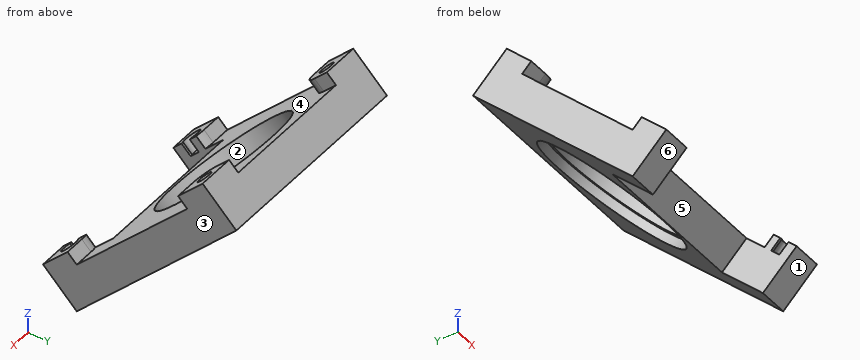
```python
from build123d import *
from OCP.BRepAlgoAPI import BRepAlgoAPI_Cut
from OCP.TopTools import TopTools_ListOfShape

# Parameters (mm, degrees)
SKETCH3_W               = 37
SKETCH3_H               = 39
SKETCH3_R               = 12
BOSS_EXTRUDE1_DEPTH     = 4.5
SKETCH4_W               = 37
SKETCH4_H               = 39
SKETCH4_R               = 13
BOSS_EXTRUDE2_DEPTH     = 1.5
SKETCH5_R               = 1.25
BOSS_EXTRUDE4_DEPTH     = 2.238877686
CUT_EXTRUDE1_DEPTH      = 3
CUT_EXTRUDE1_DEPTH_BACK = 7.261122
SKETCH7_W               = 27
SKETCH7_H               = 10


with BuildPart() as part:
    # Sketch3 → Boss-Extrude1 (new body)
    with BuildSketch(Plane(origin=(0, -51.218608926, 51.218608926), x_dir=(1, 0, 0), z_dir=(-2.4581031654591364e-15, -0.7071067811865478, 0.7071067811865472))):
        with Locations((73.844609768, 127.312236852)):
            Rectangle(SKETCH3_W, SKETCH3_H)
        with Locations(Location((73.844609768, 131.312236852, 0), (0, 0, 270))):
            Circle(SKETCH3_R, mode=Mode.SUBTRACT)
    extrude(amount=-BOSS_EXTRUDE1_DEPTH)

    # Sketch4 → Boss-Extrude2 (add)
    with BuildSketch(Plane(origin=(0, -48.036628411, 48.036628411), x_dir=(1, 0, 0), z_dir=(2.4581031654591364e-15, 0.7071067811865478, -0.7071067811865472))):
        with Locations((73.844609768, -127.312236852)):
            Rectangle(SKETCH4_W, SKETCH4_H)
        with Locations(Location((73.844609768, -131.312236852, 0), (0, 0, 90))):
            Circle(SKETCH4_R, mode=Mode.SUBTRACT)
    extrude(amount=BOSS_EXTRUDE2_DEPTH)

    # Sketch5 → Boss-Extrude4 (add)
    # profile 1 of 4: a face of its own
    with BuildSketch(Plane(origin=(0, -51.218608926, 51.218608926), x_dir=(1, 0, 0), z_dir=(-2.386964886512496e-15, -0.7071067811865477, 0.7071067811865475))):
        with BuildLine():
            Line((92.344609768, 107.812236852), (92.344609768, 113.812236852))
            Line((92.344609768, 113.812236852), (88.844609768, 113.812236852))
            ThreePointArc((88.844609768, 113.812236852), (88.068152632, 113.710014331), (87.344609768, 113.410313064))
            Line((87.344609768, 113.410313064), (87.344609768, 111.807298734))
            Line((87.344609768, 111.807298734), (87.722178544, 111.807298734))
            ThreePointArc((87.722178544, 111.807298734), (90.344606124, 110.815542933), (87.726575779, 109.812236852))
            Line((87.726575779, 109.812236852), (87.344609768, 109.812236852))
            Line((87.344609768, 109.812236852), (87.344609768, 107.812236852))
            Line((87.344609768, 107.812236852), (92.344609768, 107.812236852))
        make_face()
    # profile 2 of 4: a face of its own
    with BuildSketch(Plane(origin=(0, -51.218608926, 51.218608926), x_dir=(1, 0, 0), z_dir=(-2.386964886512496e-15, -0.7071067811865477, 0.7071067811865475))):
        with BuildLine():
            Line((55.344609768, 107.812236852), (60.344609768, 107.812236852))
            Line((60.344609768, 107.812236852), (60.344609768, 109.812236852))
            Line((60.344609768, 109.812236852), (59.962643756, 109.812236852))
            ThreePointArc((59.962643756, 109.812236852), (57.344609768, 110.812236852), (59.962643756, 111.812236852))
            Line((59.962643756, 111.812236852), (60.344609768, 111.812236852))
            Line((60.344609768, 111.812236852), (60.344609768, 113.410313064))
            ThreePointArc((60.344609768, 113.410313064), (59.621066903, 113.710014331), (58.844609768, 113.812236852))
            Line((58.844609768, 113.812236852), (55.344609768, 113.812236852))
            Line((55.344609768, 113.812236852), (55.344609768, 107.812236852))
        make_face()
    # profile 3 of 4: a face of its own
    with BuildSketch(Plane(origin=(0, -51.218608926, 51.218608926), x_dir=(1, 0, 0), z_dir=(-2.386964886512496e-15, -0.7071067811865477, 0.7071067811865475))):
        with BuildLine():
            Line((55.344609768, 146.812236852), (55.344609768, 140.812236852))
            Line((55.344609768, 140.812236852), (58.844609768, 140.812236852))
            ThreePointArc((58.844609768, 140.812236852), (60.965930111, 141.690916509), (61.844609768, 143.812236852))
            Line((61.844609768, 143.812236852), (61.844609768, 146.812236852))
            Line((61.844609768, 146.812236852), (55.344609768, 146.812236852))
        make_face()
        with Locations(Location((58.844609768, 143.812236852, 0), (0, 0, 90))):
            Circle(SKETCH5_R, mode=Mode.SUBTRACT)
    # profile 4 of 4: a face of its own
    with BuildSketch(Plane(origin=(0, -51.218608926, 51.218608926), x_dir=(1, 0, 0), z_dir=(-2.386964886512496e-15, -0.7071067811865477, 0.7071067811865475))):
        with BuildLine():
            Line((92.344609768, 146.812236852), (85.844609768, 146.812236852))
            Line((85.844609768, 146.812236852), (85.844609768, 143.812236852))
            ThreePointArc((85.844609768, 143.812236852), (86.723289424, 141.690916509), (88.844609768, 140.812236852))
            Line((88.844609768, 140.812236852), (92.344609768, 140.812236852))
            Line((92.344609768, 140.812236852), (92.344609768, 146.812236852))
        make_face()
        with Locations(Location((88.844609768, 143.812236852, 0), (0, 0, 90))):
            Circle(SKETCH5_R, mode=Mode.SUBTRACT)
    extrude(amount=BOSS_EXTRUDE4_DEPTH)


with BuildPart() as cut_extrude1_tool:
    # Sketch7 → Cut-Extrude1 (new, two sides: drawn at the far end of the back side and taken through both)
    with BuildSketch(Plane(origin=(0, -46.084220099, 46.084220099), x_dir=(1, 0, 0), z_dir=(0, 0.7071067811865502, -0.7071067811865449)).offset(-CUT_EXTRUDE1_DEPTH_BACK)):
        with Locations((73.844609768, -112.812236852)):
            Rectangle(SKETCH7_W, SKETCH7_H)
    extrude(amount=CUT_EXTRUDE1_DEPTH + CUT_EXTRUDE1_DEPTH_BACK)


with BuildPart() as part_1:
    add(part.part)

    # Cut-Extrude1: cut by cut_extrude1_tool, with a tolerance
    cut_extrude1_stock = TopTools_ListOfShape()
    cut_extrude1_stock.Append(part_1.part.wrapped)
    cut_extrude1_tools = TopTools_ListOfShape()
    cut_extrude1_tools.Append(cut_extrude1_tool.part.wrapped)
    cut_extrude1_cut = BRepAlgoAPI_Cut()
    cut_extrude1_cut.SetArguments(cut_extrude1_stock)
    cut_extrude1_cut.SetTools(cut_extrude1_tools)
    cut_extrude1_cut.SetFuzzyValue(0.00001)
    cut_extrude1_cut.Build()
    add(Compound.cast(cut_extrude1_cut.Shape()).solids(), mode=Mode.REPLACE)


solid = part_1.part
```
Source: CAD feature listing. Evaluate the final solid. Frame: model axes, mm. Face numbers are marked on the shaded views. A direction names the side the tool comes from. Coordinates: 2 decimals unless noted, no trailing zeros. Loops run counter-clockwise (first coordinate to the right, second up) from the corner with the lowest first, then second, coordinate; pieces in that order, holes last. Notation, with made-up numbers: M 32,8 L 74,8 A25 cw 74,30 Z; hole C 27.5,10.5 d10. An arc over 180 degrees is marked long. Put each result on its own line as item: value. Start each with the question number.
1) Reachability of the marked faces 5 and 6 from +Z, -Z, +X, -X, +Y, -Y: full face, straight path, thin tool, end or side. Return the list, or none.
2) Cut plane D-D on x = 89.5. Return the cut outline in (y, z) (1 decimal), then the cut area to 3 significant figures.
3) Pull-direction query (X, two-part tool) for the marked faces 1, 2, 3 and 4; classes: pulls with the +X half, pulls with the -X half, needs draft (parallel to the pull), parting line crosses it, or undercut.
4) Cut plane B-B on z = 125.5. Return the cut outline in (x, y).
5) Contact query for flat-ended pins moving along their axis: pin 1 Ø3 at (x, z) = (71, 151) entering from -Y; pin 2 Ø12 at (x, z) = (77, 147) entering from -Y; pin 3 Ø8 at (x, z) = (84.5, 146.5) entering from -Y. Output: stop coordinate, or through.
6) Ray query, L1, parallel to X at y = 26.5, z = 126; L2, parallel to X at y = 38, z = 133; L3, parallel to Y at x = 57, z = 134. Return the intervals inside material, ascending. Write a range as from..to.
7) Cut plane C-C on y = 30.5. Return the cut outline in (x, z).
8) Cut plane A-A on x = 75. Return the cut outline in (y, z).
The answers:
1. face 5: -Z, -Y
1. face 6: -Z, +X, -X, -Y
2. outline: M 23.4,129 L 29.3,123.2 L 56.8,150.8 L 51,156.6 L 49.6,155.2 L 51.2,153.7 L 49.7,152.2 L 48.1,153.7 L 46.8,152.4 L 48.4,150.8 L 29.3,131.7 L 27.7,133.3 L 26.5,132.1 L 28.1,130.5 L 26.2,128.6 L 24.6,130.2 Z
2. area: 250 mm²
3. face 1: needs draft
3. face 2: undercut
3. face 3: pulls with the +X half
3. face 4: undercut
4. outline: M 55.34,26.97 L 60.34,26.97 L 60.34,31.55 L 55.34,31.55 Z; M 87.34,26.97 L 92.34,26.97 L 92.34,31.55 L 87.34,31.55 Z
5. pin 1: stops at y = 49.67
5. pin 2: stops at y = 47.84
5. pin 3: stops at y = 40.24
6. L1: x = 55.34..60.34, 87.34..92.34
6. L2: x = 55.34..66.04, 81.65..92.34
6. L3: y = 31.56..40.05
7. outline: M 55.34,124.45 L 60.34,124.45 L 60.34,132.94 L 55.34,132.94 Z; M 87.34,124.45 L 92.34,124.45 L 92.34,132.94 L 87.34,132.94 Z
8. outline: M 32.09,134.52 L 36.33,130.28 L 36.72,130.67 L 35.66,131.73 L 36.37,132.44 L 33.19,135.62 Z; M 50.08,152.52 L 53.26,149.33 L 53.97,150.04 L 55.03,148.98 L 56.84,150.79 L 52.59,155.03 Z
